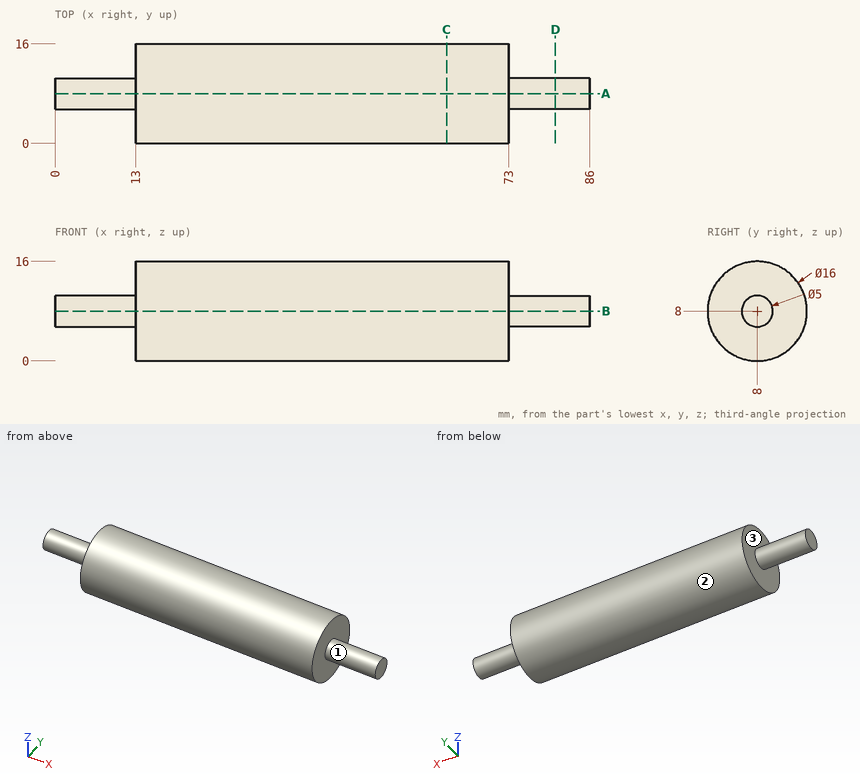
Part print with two shaded views. Sizes in mm from the minimum x, y, z corner. A direction names the side the tool comes from. Round coordinates to 2 decimals unless told otherwise and drop trailing zeros. Order: outer loops, then holes, each group sorted by start corner. A loop starts at its lowest first (then second) coordinate and runs counter-clockwise, first axis right, second up. Notation, with made-up numbers: (20.25, -2.75) - (73.25, -2.75) arc R26 ccw to (73.25, 13.25) - close; hole circle Ø2 at (-37.5, 64.25). An arc over 180 degrees is marked (long way). Return JSON: item names as keys, results as strings.
(1) Wall check: probe 1 along X at (y, z) = (3.5, 9.25); probe 2 along Y at (x, z) = (46, 7.5); probe 3 along Y at (x, z) = (34, 14.75). Give the ranges that are in metal, low to high. Write a range as from..to.
Answer key:
{"probe 1": "x = 13..73", "probe 2": "y = 0.02..15.98", "probe 3": "y = 3.71..12.29"}
(2) Cut at C-C (x = 63). Give the cut face in (y, z), then the cut area to 3 significant figures.
Answer key:
{"outline": "circle Ø16 at (8, 8)", "area": "201 mm^2"}
(3) Cut at D-D (x = 80.5). Give the cut face in (y, z).
Answer key:
{"outline": "circle Ø5 at (8, 8)"}
(4) Tool access for the marked faces 1, 2 and 3: list every direction of +Z, -Z, +X, -X, +Y, -Y with a clear straight run to the whole face (end or side of a thin tool).
Answer key:
{"face 1": "+X", "face 2": "+X, -X", "face 3": "-X"}
(5) Cut at A-A (y = 8). Give the cut face in (x, z), then the cut area to 3 significant figures.
Answer key:
{"outline": "(0, 5.5) - (13, 5.5) - (13, 0) - (73, 0) - (73, 5.5) - (86, 5.5) - (86, 10.5) - (73, 10.5) - (73, 16) - (13, 16) - (13, 10.5) - (0, 10.5) - close", "area": "1,090 mm^2"}
(6) Pin check, flat tips, straight feed: pin 1 Ø2 at (x, z) = (55.5, 4) entering from +Y; pin 2 Ø2 at (x, z) = (28.5, 13.5) entering from +Y; pin 3 Ø5 at (x, y) = (36, 12.5) entering from -Z. Stop position of each tip, or through.
Answer key:
{"pin 1": "stops at y = 15.42", "pin 2": "stops at y = 14.61", "pin 3": "stops at z = 0.25"}
